Could you check a few things on this model? Use its own coordinates, in mm. A direction names the side the tool comes from. Coordinates: 2 decimals unless noted, no trailing zeros. Order: outer loops, then holes, each group sorted by start corner. A loop starts at its lowest first (then second) coordinate and runs counter-clockwise, first axis right, second up. Notation, with made-up numbers: M 80.5,53 L 85.5,53 A23 ccw 85.5,77 Z; hole C -12,5.5 d11. An arc over 180 degrees is marked long. Put each result on its own line as item: value. Start each with the question number.
```python
from build123d import *

# Parameters (mm, degrees)
F0_W     = 6.8689025939
F0_H     = 6.8689035252
F0_W_2   = 12.8473937511
F0_H_2   = 32.5636891648
F2_R     = 22.3587464381
F3_DEPTH = 7.62
F5_DEPTH = 6.35


with BuildPart() as f1:
    # F0 (on Front) → F1 (revolve)
    with BuildSketch(Plane.XZ):
        Polygon((0, 48.5911294818), (0, 39.43259269), (12.8473937511, 39.43259269), (26.5851970762, 39.43259269), (26.5851970762, 48.5911294818), align=None)
        with Locations((16.2818450481, 3.4344517626)):
            Rectangle(F0_W, F0_H)
        with Locations((6.4236968756, 23.1507481076)):
            Rectangle(F0_W_2, F0_H_2)
        with Locations((6.4236968756, 3.4344517626)):
            Rectangle(F0_W_2, F0_H)
    revolve(axis=Axis((0, 0, 19.716296345), (0, 0, 1)))

    # F2 (on face) → F3 (cut)
    with BuildSketch(Plane.XY.offset(48.5911294818)):
        Circle(F2_R)
    extrude(amount=-F3_DEPTH, mode=Mode.SUBTRACT)

    # F4 (on face) → F5 (cut)
    with BuildSketch(Plane.XY.offset(48.5911294818)):
        with BuildLine():
            ThreePointArc((-3.0514306297, 17.3055230542), (0, 17.5724886419), (3.0514306297, 17.3055230542))
            Line((3.0514306297, 17.3055230542), (5.4403788798, 30.8539218326))
            ThreePointArc((5.4403788798, 30.8539218326), (0, 31.3298933099), (-5.4403788798, 30.8539218326))
            Line((-5.4403788798, 30.8539218326), (-3.0514306297, 17.3055230542))
        make_face()
        with BuildLine():
            ThreePointArc((-16.5127379056, 6.0101450839), (-15.2182215716, 8.7862443209), (-13.4613072759, 11.2953779703))
            Line((-13.4613072759, 11.2953779703), (-24.0000906736, 20.1384672324))
            ThreePointArc((-24.0000906736, 20.1384672324), (-27.1324835042, 15.664946655), (-29.4404695533, 10.7154546002))
            Line((-29.4404695533, 10.7154546002), (-16.5127379056, 6.0101450839))
        make_face()
        with BuildLine():
            ThreePointArc((-13.4613072759, -11.2953779703), (-15.2182215716, -8.7862443209), (-16.5127379056, -6.0101450839))
            Line((-16.5127379056, -6.0101450839), (-29.4404695533, -10.7154546002))
            ThreePointArc((-29.4404695533, -10.7154546002), (-27.1324835042, -15.664946655), (-24.0000906736, -20.1384672324))
            Line((-24.0000906736, -20.1384672324), (-13.4613072759, -11.2953779703))
        make_face()
        with BuildLine():
            ThreePointArc((3.0514306297, -17.3055230542), (0, -17.5724886419), (-3.0514306297, -17.3055230542))
            Line((-3.0514306297, -17.3055230542), (-5.4403788798, -30.8539218326))
            ThreePointArc((-5.4403788798, -30.8539218326), (0, -31.3298933099), (5.4403788798, -30.8539218326))
            Line((5.4403788798, -30.8539218326), (3.0514306297, -17.3055230542))
        make_face()
        with BuildLine():
            ThreePointArc((16.5127379056, -6.0101450839), (15.2182215716, -8.7862443209), (13.4613072759, -11.2953779703))
            Line((13.4613072759, -11.2953779703), (24.0000906736, -20.1384672324))
            ThreePointArc((24.0000906736, -20.1384672324), (27.1324835042, -15.664946655), (29.4404695533, -10.7154546002))
            Line((29.4404695533, -10.7154546002), (16.5127379056, -6.0101450839))
        make_face()
        with BuildLine():
            ThreePointArc((13.4613072759, 11.2953779703), (15.2182215716, 8.7862443209), (16.5127379056, 6.0101450839))
            Line((16.5127379056, 6.0101450839), (29.4404695533, 10.7154546002))
            ThreePointArc((29.4404695533, 10.7154546002), (27.1324835042, 15.664946655), (24.0000906736, 20.1384672324))
            Line((24.0000906736, 20.1384672324), (13.4613072759, 11.2953779703))
        make_face()
    extrude(amount=-F5_DEPTH, mode=Mode.SUBTRACT)


solid = f1.part
```
Item 1: I need wall thicknesses on probe 1 along Z at (x, y) = (-10, -14); probe 2 along X at (y, z) = (0, 45.25); probe 3 along Z at (x, y) = (5.5, 10). Which ranges of each line are inside material? Lowest first, please.
Item 2: If we mould it in two halves opening along Y, with no side actions, what happens to faces 1 (the flat face through (21, -12, 42.241)), 2 (the cylindrical face through (-2.79, -12.54, 23.38)), 3 (the flat face through (12, -20, 48.591))? For each: released by +Y, released by -Y, zero draft, split by the parting line, or undercut.
Item 3: For faces 4 (the flat face through (0, -24, 42.241)), 5 (the flat face through (-18.72, 15.71, 45.46)), 6 (the flat face through (-23.02, 8.38, 45.46)), 7 (the flat face through (-13, 0, 6.869)), which set-ups out of +Z, -Z, +X, -X, +Y, -Y let a thin tool reach every point of the face, with its end or its side?
Item 4: If we section it at C-C on x = 0: Write out the boundary of the cut face in (y, z).
Item 5: If we section it at B-B on y = 0: Write out the boundary of the cut face in (x, z), then the cut area to 3 significant figures.
Item 6: If we section it at A-A on x = -14.5: Write out the boundary of the cut face in (y, z).
Item 7: For pin 1 Ø12 at (y, z) = (8.5, 20.5) entering from -X; pin 2 Ø1.5 at (x, y) = (12.5, 17.5) entering from +Z; pin 3 Ø8 at (x, z) = (-15.5, 6.5) entering from -Y, each with a flat end and sliding along its axis, tell me the tip position at first contact or that it passes through.
Item 8: If we section it at D-D on z = 5: Write out the boundary of the cut face in (x, y).
Geometry check:
1. probe 1: z = 0 to 6.87, 39.43 to 40.97
1. probe 2: x = -26.59 to -22.36, 22.36 to 26.59
1. probe 3: z = 0 to 40.97
2. face 1: undercut
2. face 2: split by the parting line
2. face 3: zero draft
3. face 4: +Z, -Y
3. face 5: +Z, -X
3. face 6: +Z, +Y
3. face 7: none
4. outline: M -26.59,39.43 L -12.85,39.43 L -12.85,6.87 L -19.72,6.87 L -19.72,0 L 19.72,0 L 19.72,6.87 L 12.85,6.87 L 12.85,39.43 L 26.59,39.43 L 26.59,42.24 L 22.36,42.24 L 22.36,40.97 L -22.36,40.97 L -22.36,42.24 L -26.59,42.24 Z
5. outline: M -26.59,39.43 L -12.85,39.43 L -12.85,6.87 L -19.72,6.87 L -19.72,0 L 19.72,0 L 19.72,6.87 L 12.85,6.87 L 12.85,39.43 L 26.59,39.43 L 26.59,48.59 L 22.36,48.59 L 22.36,40.97 L -22.36,40.97 L -22.36,48.59 L -26.59,48.59 Z
5. area: 1,250 mm²
6. outline: M -22.28,39.43 L 22.28,39.43 L 22.28,48.59 L 17.02,48.59 L 17.02,40.97 L -17.02,40.97 L -17.02,48.59 L -22.28,48.59 Z; M -13.36,0 L 13.36,0 L 13.36,6.87 L -13.36,6.87 Z
7. pin 1: stops at x = -12.6
7. pin 2: stops at z = 40.97
7. pin 3: stops at y = -16.02
8. outline: C 0,0 d39.43
